```python
from build123d import *

# Parameters (mm, degrees)
SKETCH_1_W          = 67.09
SKETCH_1_H          = 50
EXTRUDE_1_DEPTH     = 10
SKETCH_2_R          = 2.5
SKETCH_2_R_2        = 1.5
CUT_EXTRUDE_1_DEPTH = 85.267835501
SKETCH_3_R          = 1.5
CUT_EXTRUDE_2_DEPTH = 85.267835592


with BuildPart() as part:
    # 草图1 → 凸台-拉伸1 (new body)
    with BuildSketch(Plane.XY):
        with Locations((33.545, 25)):
            Rectangle(SKETCH_1_W, SKETCH_1_H)
        with BuildLine():
            Line((11, 45), (56.09, 45))
            ThreePointArc((56.09, 45), (60.332640687, 43.242640687), (62.09, 39))
            Line((62.09, 39), (62.09, 11))
            ThreePointArc((62.09, 11), (60.332640687, 6.757359313), (56.09, 5))
            Line((56.09, 5), (11, 5))
            ThreePointArc((11, 5), (6.757359313, 6.757359313), (5, 11))
            Line((5, 11), (5, 39))
            ThreePointArc((5, 39), (6.757359313, 43.242640687), (11, 45))
        make_face(mode=Mode.SUBTRACT)
    extrude(amount=EXTRUDE_1_DEPTH)

    # 草图2 → 切除-拉伸1 (cut, through all)
    with BuildSketch(Plane.ZY):
        with Locations((5, 42)):
            Circle(SKETCH_2_R)
        with Locations((5, 8)):
            Circle(SKETCH_2_R)
        with Locations((5, 25)):
            Circle(SKETCH_2_R_2)
    extrude(amount=-CUT_EXTRUDE_1_DEPTH, mode=Mode.SUBTRACT)

    # 草图3 → 切除-拉伸2 (cut, through all)
    with BuildSketch(Plane.XZ):
        with Locations(Location((33.545, 5, 0), (0, 0, 270))):
            Circle(SKETCH_3_R)
    extrude(amount=-CUT_EXTRUDE_2_DEPTH, mode=Mode.SUBTRACT)


solid = part.part
```
Check sheet for the modelled part. Datum: model origin and axes. Units: mm. A direction names the side the tool comes from. Coordinates: 2 decimals unless noted, no trailing zeros. Order: outer loops, then holes, each group sorted by start corner. A loop starts at its lowest first (then second) coordinate and runs counter-clockwise, first axis right, second up. Notation, with made-up numbers: (24.5, 60.5) -> (30.5, 60.5) arc R23 ccw to (30.5, 76.5) -> close; hole circle Ø4 at (54.25, -1). An arc over 180 degrees is marked (long way). Write each question's results on one line, items separated by ' | '. Start each with the question number.
1) Section check D-D (y = 8). Enter the section's corners in (x, z).
2) Set-up check for faces 1 (the face through (2.465, 26.487, 4.805)), 2 (the face through (62.09, 25, 3)): record each of +Z, -Z, +X, -X, +Y, -Y from which the full face is reachable in a straight line by a thin tool's end or side.
3) Section check C-C (z = 1.5). Enter the section's corners in (x, y), and give its area (3 significant figures).
4) Section check B-B (x = 15). Enter the section's corners in (y, z).
5) Section check A-A (y = 28). Enter the section's corners in (x, z).
6) Material ranges on line 1 along Y through (x, z) = (62.75, 5); line 2 along Y through (x, z) = (19, 9); line 3 along X through (y, z) = (22, 4.5), recorded low to high.
7) Draft check along Z on faces 3 (the face through (63.68, 44.48, 4.67)), 4 (the face through (5, 25, 3)), 5 (the face through (33, 3, 0)). Enter one of: pulls with the +Z half, pulls with the -Z half, needs draft (parallel to the pull), parting line crosses it, or undercut.
8) Depth check by flat-ended pin: pin 1 (2.5 mm diameter, centred on y = 25, z = 5, fed in from +X). Enter the tip coordinate at first touch or a pass-through.
Checked values:
1) outline: (0, 0) -> (5.8, 0) -> (5.8, 2.5) -> (0, 2.5) -> close; (0, 7.5) -> (5.8, 7.5) -> (5.8, 10) -> (0, 10) -> close; (61.29, 0) -> (67.09, 0) -> (67.09, 2.5) -> (61.29, 2.5) -> close; (61.29, 7.5) -> (67.09, 7.5) -> (67.09, 10) -> (61.29, 10) -> close
2) face 1: +X, -X | face 2: +Z, -Z
3) outline: (0, 0) -> (67.09, 0) -> (67.09, 50) -> (0, 50) -> close; hole (5, 11) arc R6 ccw to (11, 5) -> (56.09, 5) arc R6 ccw to (62.09, 11) -> (62.09, 39) arc R6 ccw to (56.09, 45) -> (11, 45) arc R6 ccw to (5, 39) -> close | area: 1,100 mm²
4) outline: (0, 0) -> (5, 0) -> (5, 10) -> (0, 10) -> close; (45, 0) -> (50, 0) -> (50, 10) -> (45, 10) -> close
5) outline: (0, 0) -> (5, 0) -> (5, 10) -> (0, 10) -> close; (62.09, 0) -> (67.09, 0) -> (67.09, 10) -> (62.09, 10) -> close
6) line 1: 0 to 5.5, 10.5 to 23.5, 26.5 to 39.5, 44.5 to 50 | line 2: 0 to 5, 45 to 50 | line 3: 0 to 5, 62.09 to 67.09
7) face 3: undercut | face 4: needs draft | face 5: pulls with the -Z half
8) pin 1: through
